For this review, use the dimensioned drawing (mm, ordinates from the lowest corner) and the shaded views. A direction names the side the tool comes from. Give positions to 0.01 mm unless a question says otherwise; leave off trailing zeros. Write each loop counter-clockwise with the first axis right and the second up, starting at its lowest first coordinate (ties: lowest second). Pieces come first, ordered by that corner, then holes. Notation, with made-up numbers: (49.5, 44) -> (91.5, 44) arc R14 ccw to (91.5, 64) -> close; hole circle Ø10 at (15.25, 36). An arc over 180 degrees is marked (long way). Answer as CSV lines item,"result".
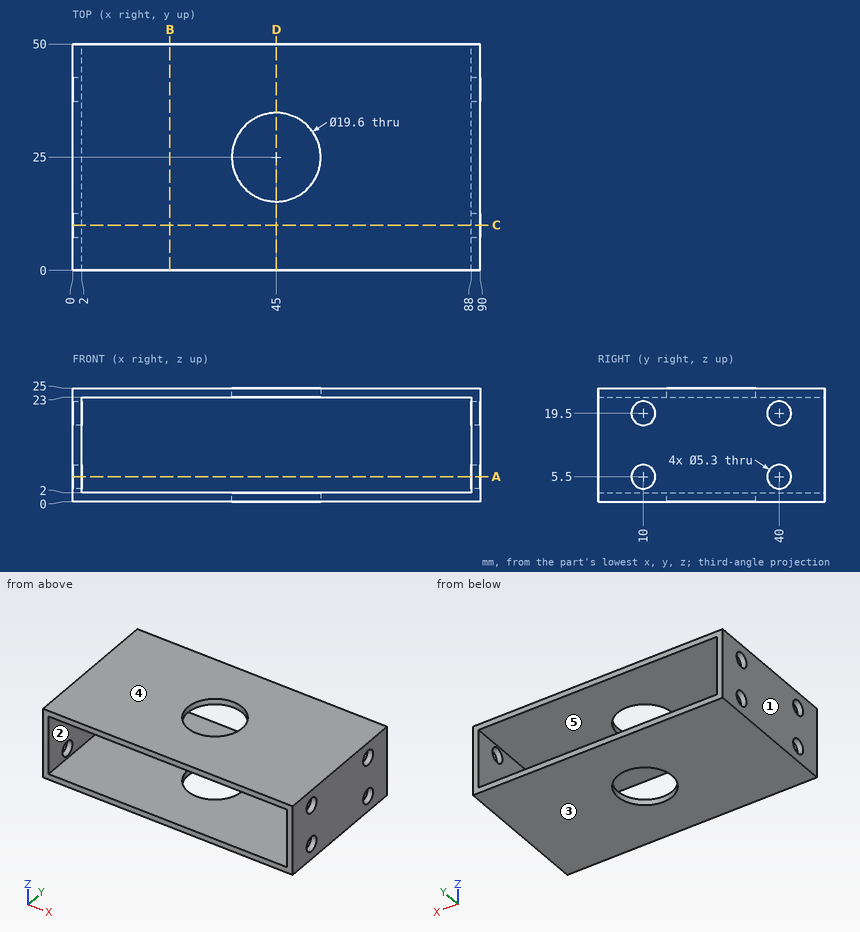
Q1. Add section D-D (x = 45). Write out the cut boundary in (y, z).
Answer block:
outline,"(0, 0) -> (15.2, 0) -> (15.2, 2) -> (0, 2) -> close; (0, 23) -> (15.2, 23) -> (15.2, 25) -> (0, 25) -> close; (34.8, 0) -> (50, 0) -> (50, 2) -> (34.8, 2) -> close; (34.8, 23) -> (50, 23) -> (50, 25) -> (34.8, 25) -> close"
Q2. Draft analysis for pull direction Z (two halves, no side actions). For the marked faces 1, 2 and 3, state which applies: released by +Z, released by -Z, zero draft, split by the parting line, or undercut.
Answer block:
face 1,"zero draft"
face 2,"undercut"
face 3,"released by -Z"
Q3. Add section A-A (z = 5.5). Write out the cut boundary in (x, y), plus the area to 3 significant figures.
Answer block:
outline,"(0, 0) -> (2, 0) -> (2, 7.35) -> (0, 7.35) -> close; (0, 12.65) -> (2, 12.65) -> (2, 37.35) -> (0, 37.35) -> close; (0, 42.65) -> (2, 42.65) -> (2, 50) -> (0, 50) -> close; (88, 0) -> (90, 0) -> (90, 7.35) -> (88, 7.35) -> close; (88, 12.65) -> (90, 12.65) -> (90, 37.35) -> (88, 37.35) -> close; (88, 42.65) -> (90, 42.65) -> (90, 50) -> (88, 50) -> close"
area,"158 mm2"
Q4. Add section B-B (x = 21.5). Write out the cut boundary in (y, z).
Answer block:
outline,"(0, 0) -> (50, 0) -> (50, 2) -> (0, 2) -> close; (0, 23) -> (50, 23) -> (50, 25) -> (0, 25) -> close"
Q5. To check wall thickness, follow probe 1 along Y at (x, z) = (88.4, 5.5); probe 2 along Z at (x, y) = (13, 43.5); probe 3 along X at (y, z) = (12, 12.5). State the ranges of each line that lie inside material, in increasing order. Write a range as [from, to].
Answer block:
probe 1,"y = [0, 7.35], [12.65, 37.35], [42.65, 50]"
probe 2,"z = [0, 2], [23, 25]"
probe 3,"x = [0, 2], [88, 90]"
Q6. Add section C-C (y = 10). Write out the cut boundary in (x, z), plus the area to 3 significant figures.
Answer block:
outline,"(0, 0) -> (90, 0) -> (90, 2.85) -> (88, 2.85) -> (88, 2) -> (2, 2) -> (2, 2.85) -> (0, 2.85) -> close; (0, 8.15) -> (2, 8.15) -> (2, 16.85) -> (0, 16.85) -> close; (0, 22.15) -> (2, 22.15) -> (2, 23) -> (88, 23) -> (88, 22.15) -> (90, 22.15) -> (90, 25) -> (0, 25) -> close; (88, 8.15) -> (90, 8.15) -> (90, 16.85) -> (88, 16.85) -> close"
area,"402 mm2"
Q7. Clearance check with a flat-ended pin moving along its axis: pin 1 (3 mm diameter, centred on y = 40, z = 19.5, fed in from -X). State where the tip first meets the part, or that it passes through.
Answer block:
pin 1,"passes through"
Q8. For the marked faces 4 and 5, list the 3-axis set-ups (+Z, -Z, +X, -X, +Y, -Y) from which the entire face can be reached by the end or side of a thin tool; tool diameter is ignored.
Answer block:
face 4,"+Z, +X, -X, +Y, -Y"
face 5,"+Y, -Y"
